Here's how the part is built. I have some questions about the finished solid (model axes, mm). A direction names the side the tool comes from. Give positions to 0.01 mm unless a question says otherwise; leave off trailing zeros. Write each loop counter-clockwise with the first axis right and the second up, starting at its lowest first coordinate (ties: lowest second). Pieces come first, ordered by that corner, then holes. Notation, with made-up numbers: (6, 39) -> (10, 39) arc R23 cw to (10, 55) -> close; hole circle Ø4 at (20.5, -32). An arc over 180 degrees is marked (long way). Put each result on its own line as item: value. Start each with the question number.
from build123d import *

# Parameters (mm, degrees)
SKETCH1_R           = 2.8448
SKETCH1_R_2         = 1.27
BOSS_EXTRUDE1_DEPTH = 4.4704
SKETCH2_R           = 3.2512
CUT_EXTRUDE1_DEPTH  = 1.143
SKETCH3_R           = 1.9939
CUT_EXTRUDE2_DEPTH  = 1.016
CUT_EXTRUDE3_DEPTH  = 3.683
SCALE1_SCALE        = 0.6


with BuildPart() as part:
    # Sketch1 → Boss-Extrude1 (new body)
    with BuildSketch(Plane(origin=(0, 0, 0), x_dir=(0, 0, -1), z_dir=(1, 0, 0))):
        with BuildLine():
            Line((0, 4.000000128), (27.94, 4.000000128))
            ThreePointArc((27.94, 4.000000128), (31.940000128, 0), (27.94, -4.000000128))
            Line((27.94, -4.000000128), (0, -4.000000128))
            ThreePointArc((0, -4.000000128), (-4.000000128, 0), (0, 4.000000128))
        make_face()
        Circle(SKETCH1_R, mode=Mode.SUBTRACT)
        with Locations((27.94, 0)):
            Circle(SKETCH1_R_2, mode=Mode.SUBTRACT)
    extrude(amount=BOSS_EXTRUDE1_DEPTH)

    # Sketch2 → Cut-Extrude1 (cut)
    with BuildSketch(Plane(origin=(4.4704, 0, 0), x_dir=(0, 0, -1), z_dir=(1, 0, 0))):
        Circle(SKETCH2_R)
    extrude(amount=-CUT_EXTRUDE1_DEPTH, mode=Mode.SUBTRACT)

    # Sketch3 → Cut-Extrude2 (cut)
    with BuildSketch(Plane(origin=(4.4704, 0, 0), x_dir=(0, 0, -1), z_dir=(1, 0, 0))):
        with Locations((27.94, 0)):
            Circle(SKETCH3_R)
    extrude(amount=-CUT_EXTRUDE2_DEPTH, mode=Mode.SUBTRACT)

    # Sketch4 → Cut-Extrude3 (cut)
    with BuildSketch(Plane(origin=(4.4704, 0, 0), x_dir=(0, 0, -1), z_dir=(1, 0, 0))):
        with BuildLine():
            Line((7.0259921, 2.54), (21.9611921, 2.54))
            ThreePointArc((21.9611921, 2.54), (24.5011921, 0), (21.9611921, -2.54))
            Line((21.9611921, -2.54), (7.0259921, -2.54))
            ThreePointArc((7.0259921, -2.54), (4.4859921, 0), (7.0259921, 2.54))
        make_face()
    extrude(amount=-CUT_EXTRUDE3_DEPTH, mode=Mode.SUBTRACT)


with BuildPart() as part_1:
    # Scale1: scaled about (2.002001382, 0, -15.510759507)
    add(part.part.scale(SCALE1_SCALE).moved(Location((0.800800553, 0, -6.204303803))))


solid = part_1.part
1) Which directions (+Z, -Z, +X, -X, +Y, -Y) give clear straight access to the entire face, cutting with the end or side of a thin tool? Please do faces 4 (the flat face through (2, -1.524, -15)), 5 (the cylindrical face through (1.823, 0.034, -22.207)).
2) I want a section at B-B, the plane y = 0. Write out the boundary of the cut face in (x, z).
3) I want a section at A-A, the plane x = 2.3. Write out the boundary of the cut face in (y, z).
4) I'm going to push flat-ended pins straight in: pin 1 Ø1.5 at (y, z) = (-0.5, -12) entering from +X; pin 2 Ø2 at (y, z) = (0, -22.97) entering from +X; pin 3 Ø1 at (x, y) = (3, -1.5) entering from -Z. Where does each tip first touch, or does it pass through?
5) Thinking about a two-plate mould opening in Y: for faces 1 (the cylindrical face through (2.123, -0.053, -3.805)), 2 (the cylindrical face through (3.18, 0.36, -24.11)), 3 (the flat face through (3.483, -2, -17)), which applies, released by +Y, released by -Y, zero draft, split by the parting line, or undercut?
6) I want a section at D-D, the plane y = -1. Write out the boundary of the cut face in (x, z).
7) I need wall thicknesses on probe 1 along Z at (x, y) = (2.1, 0); probe 2 along Y at (x, z) = (2.9, -17.5); probe 3 along Z at (x, y) = (2, 0.8). Which ranges of each line are inside material? Lowest first, please.
8) I want a section at C-C, the plane z = -13.5. Write out the boundary of the cut face in (x, y), and give its area (3 significant figures).
Established:
1. face 4: +X
1. face 5: +X, -X
2. outline: (0.8, -25.37) -> (3.48, -25.37) -> (3.48, -24.16) -> (2.87, -24.16) -> (2.87, -23.73) -> (0.8, -23.73) -> close; (0.8, -22.21) -> (2.87, -22.21) -> (2.87, -21.77) -> (3.48, -21.77) -> (3.48, -20.91) -> (1.27, -20.91) -> (1.27, -8.9) -> (3.48, -8.9) -> (3.48, -8.16) -> (2.8, -8.16) -> (2.8, -7.91) -> (0.8, -7.91) -> close; (0.8, -4.5) -> (2.8, -4.5) -> (2.8, -4.25) -> (3.48, -4.25) -> (3.48, -3.8) -> (0.8, -3.8) -> close
3. outline: (-2.4, -22.97) arc R2.4 ccw to (2.4, -22.97) -> (2.4, -6.2) arc R2.4 ccw to (-2.4, -6.2) -> close; hole circle Ø3.41 at (0, -6.2); hole (-1.52, -19.38) arc R1.52 ccw to (1.52, -19.38) -> (1.52, -10.42) arc R1.52 ccw to (-1.52, -10.42) -> close; hole circle Ø1.52 at (0, -22.97)
4. pin 1: stops at x = 1.27
4. pin 2: stops at x = 2.87
4. pin 3: stops at z = -25.15
5. face 1: split by the parting line
5. face 2: undercut
5. face 3: zero draft
6. outline: (0.8, -25.15) -> (3.48, -25.15) -> (3.48, -23.62) -> (2.87, -23.62) -> (2.87, -22.31) -> (3.48, -22.31) -> (3.48, -20.53) -> (1.27, -20.53) -> (1.27, -9.27) -> (3.48, -9.27) -> (3.48, -7.88) -> (2.8, -7.88) -> (2.8, -7.59) -> (0.8, -7.59) -> close; (0.8, -4.82) -> (2.8, -4.82) -> (2.8, -4.53) -> (3.48, -4.53) -> (3.48, -4.02) -> (0.8, -4.02) -> close
7. probe 1: z = -25.37 to -23.73, -22.21 to -20.91, -8.9 to -7.91, -4.5 to -3.8
7. probe 2: y = -2.4 to -1.52, 1.52 to 2.4
7. probe 3: z = -25.23 to -20.68, -9.12 to -7.71, -4.7 to -3.94
8. outline: (0.8, -2.4) -> (3.48, -2.4) -> (3.48, -1.52) -> (1.27, -1.52) -> (1.27, 1.52) -> (3.48, 1.52) -> (3.48, 2.4) -> (0.8, 2.4) -> close
8. area: 6.14 mm2
